Read the model definition and answer for the solid it produces. Units are mm, in the model's axes. Face numbers are marked on the shaded views. A direction names the side the tool comes from. Give positions to 0.01 mm unless a question says otherwise; leave off trailing zeros. Write each loop counter-clockwise with the first axis right and the second up, starting at its lowest first coordinate (ties: lowest second). Pieces come first, ordered by that corner, then holes. Notation, with made-up numbers: M 1,-38.75 L 48,-38.75 A33 cw 48,-2.75 Z; hole C 67.5,2.5 d3. An arc over 180 degrees is marked long. Use a Markdown table: item, result. Add a question column.
Item 1: The mould has two halves that part along X. Classify the marked faces 1, 2, 3 and 4: pulls with the +X half, pulls with the -X half, needs draft (parallel to the pull), parting line crosses it, or undercut.
Item 2: Given P1, Ø6, axis at x = 3, y = 3, coming from the -Z side; P2, Ø4, axis at y = 5, z = 21.5, coming from the -X side; P3, Ø4, axis at y = 3.5, z = 21, coming from the +X side; P4, Ø11.5, axis at x = 20, z = 16, coming from the +Y side, each flat-ended and moving along its own axis, determine where each tip first touches the part or whether it passes through.
Item 3: A cutting plane is placed at A-A on y = 12. Determine the outline of the cut face in (x, z).
Item 4: For the marked faces 5, 6 and 7, determine the directions among +Z, -Z, +X, -X, +Y, -Y from which every point of the face is accessible in a straight line to the end or side of a thin tool.
Item 5: A cutting plane is placed at B-B on z = 16. Determine the outline of the cut face in (x, y).
Item 6: A cutting plane is placed at C-C on x = 60. Determine the outline of the cut face in (y, z), then the cut area to 3 significant figures.
Item 7: Consider probe 1 along X at (y, z) = (12, 16); probe 2 along X at (y, z) = (6.5, 16); probe 3 along X at (y, z) = (3.75, 18.5). Determine where each line is inside the solid, lowest interval first. Write a range as [from, to].
Item 8: A cutting plane is placed at D-D on z = 7. Determine the outline of the cut face in (x, y), then the cut area to 3 significant figures.
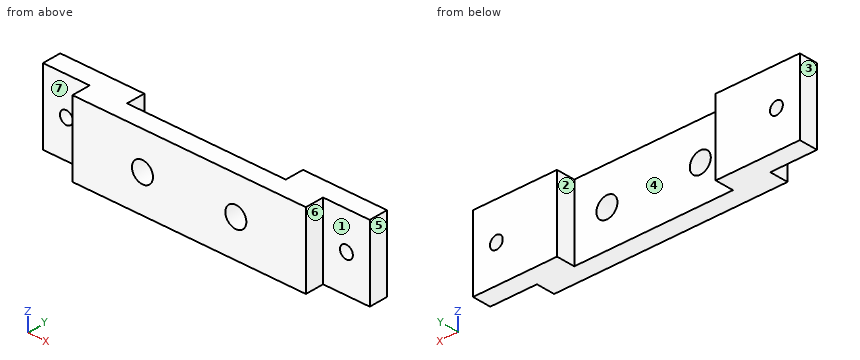
from build123d import *

# Parameters (mm, degrees)
AUFSATZ_LINEAR_AUSTRAGEN1_DEPTH  = 32
F_9_0_9_DURCHMESSER_BOHRUNG1_D   = 9
F_5_5_5_5_DURCHMESSER_BOHRUNG1_D = 5.5


with BuildPart() as part:
    # Skizze1 → Aufsatz-Linear austragen1 (new body)
    with BuildSketch(Plane.XY):
        Polygon((-70, 16), (-34, 16), (-34, 8), (34, 8), (34, 16), (70, 16), (70, 8), (50, 8), (50, 0), (-50, 0), (-50, 8), (-70, 8), align=None)
    extrude(amount=AUFSATZ_LINEAR_AUSTRAGEN1_DEPTH)

    # Ø9.0 (9) Durchmesser Bohrung1 (through all)
    with Locations(Plane(origin=(20, 8, 16), x_dir=(0, 0, 1), z_dir=(0, 1, 0))):
        with Locations((0, 0), (0, -40)):
            Hole(F_9_0_9_DURCHMESSER_BOHRUNG1_D / 2)

    # Ø5.5 (5.5) Durchmesser Bohrung1 (through all)
    with Locations(Plane(origin=(-60, 8, 16), x_dir=(-1, 0, 0), z_dir=(0, -1, 0))):
        with Locations((0, 0), (-120, 0)):
            Hole(F_5_5_5_5_DURCHMESSER_BOHRUNG1_D / 2)


solid = part.part
Filled in:
| question | item | result |
|---|---|---|
| 1 | face 1 | needs draft |
| 1 | face 2 | undercut |
| 1 | face 3 | pulls with the -X half |
| 1 | face 4 | undercut |
| 2 | P1 | z = 0 |
| 2 | P2 | x = -50 |
| 2 | P3 | x = 50 |
| 2 | P4 | y = 8 |
| 3 | outline | M -70,0 L -34,0 L -34,32 L -70,32 Z; M 34,0 L 70,0 L 70,32 L 34,32 Z; hole C -60,16 d5.5; hole C 60,16 d5.5 |
| 4 | face 5 | +Z, -Z, +X, +Y, -Y |
| 4 | face 6 | +Z, -Z, +X, -Y |
| 4 | face 7 | +Z, -Z, -X, -Y |
| 5 | outline | M -70,8 L -62.75,8 L -62.75,16 L -70,16 Z; M -57.25,8 L -50,8 L -50,0 L -24.5,0 L -24.5,8 L -34,8 L -34,16 L -57.25,16 Z; M -15.5,0 L 15.5,0 L 15.5,8 L -15.5,8 Z; M 24.5,0 L 50,0 L 50,8 L 57.25,8 L 57.25,16 L 34,16 L 34,8 L 24.5,8 Z; M 62.75,8 L 70,8 L 70,16 L 62.75,16 Z |
| 6 | outline | M 8,0 L 16,0 L 16,13.25 L 8,13.25 Z; M 8,18.75 L 16,18.75 L 16,32 L 8,32 Z |
| 6 | area | 212 mm² |
| 7 | probe 1 | [-70, -62.75], [-57.25, -34], [34, 57.25], [62.75, 70] |
| 7 | probe 2 | [-50, -24.5], [-15.5, 15.5], [24.5, 50] |
| 7 | probe 3 | [-50, -23.74], [-16.26, 16.26], [23.74, 50] |
| 8 | outline | M -70,8 L -50,8 L -50,0 L 50,0 L 50,8 L 70,8 L 70,16 L 34,16 L 34,8 L -34,8 L -34,16 L -70,16 Z |
| 8 | area | 1,380 mm² |
